Geometry: final body of the model. Coordinates: model frame, mm. A direction names the side the tool comes from. Give positions to 0.01 mm unless a question says otherwise; leave off trailing zeros. Loops run counter-clockwise (first coordinate to the right, second up) from the corner with the lowest first, then second, coordinate; pieces in that order, holes last.
1. Access query for faces 1 (the face through (0, 30, 4)), 2 (the face through (-113.606, 31.364, 8.496)), 3 (the face through (70, 22, 2)). Directions: +Z, -Z, +X, -X, +Y, -Y. A direction counts if a zero-diameter tool reaches every point of the face in a straight line with its end or side. Return the directions, or none.
2. Draft query along Y for faces 4 (the face through (-113.606, 31.364, 1.504)), 5 (the face through (-13.44, 32.25, 6.96)), 6 (the face through (2, 30, 10)), 7 (the face through (-1, 1, 2)). Return one class per face: +Y half, -Y half, draft (parallel to the pull), parting line (faces both ways), or undercut.
3. Section B-B, the plane z = 8.25. Output: boundary loops of the cut face in (x, y), then the cut area to 3 significant figures.
4. Material intervals for line 1 along X through (y, z) = (37.5, 9.5); line 2 along Y through (x, z) = (-70, 6.75); line 3 along X through (y, z) = (43, 3.25), sorted ascending.
5. First-contact query: P1, Ø1.2, axis at x = -70, y = 21.5, coming from the +Z side; P2, Ø2, axis at y = 20.5, z = 1.5, coming from the -X side; P3, Ø1.2, axis at x = -4.5, z = 2, coming from the -Y side; P4, Ø5, axis at x = 12, y = 30, coming from the -Z side. Flat tips, straight axial feed; report the tip coordinate or a pass-through.
from build123d import *

# Parameters (mm, degrees)
BOSS_EXTRUDE1_DEPTH = 10
SKETCH2_R           = 2
CUT_EXTRUDE1_DEPTH  = 8
FILLET1_R           = 5
SKETCH3_W           = 46
SKETCH3_H           = 40
CUT_EXTRUDE2_DEPTH  = 4
SKETCH4_R           = 2.672212582
CUT_EXTRUDE3_DEPTH  = 135.298175803


with BuildPart() as part:
    # Sketch1 → Boss-Extrude1 (new body)
    with BuildSketch(Plane.XY):
        with BuildLine():
            Line((0, 0), (-105, 0))
            ThreePointArc((-105, 0), (-117.249623327, 6.342822149), (-119.139622366, 20.007102889))
            Line((-119.139622366, 20.007102889), (-110.875178831, 43.345171481))
            ThreePointArc((-110.875178831, 43.345171481), (-101.737771304, 55.416038879), (-87.309141554, 60))
            Line((-87.309141554, 60), (87.309141554, 60))
            ThreePointArc((87.309141554, 60), (101.737771304, 55.416038879), (110.875178831, 43.345171481))
            Line((110.875178831, 43.345171481), (119.139622366, 20.007102889))
            ThreePointArc((119.139622366, 20.007102889), (117.249623327, 6.342822149), (105, 0))
            Line((105, 0), (0, 0))
        make_face()
    extrude(amount=BOSS_EXTRUDE1_DEPTH)

    # Sketch2 → Cut-Extrude1 (cut)
    with BuildSketch(Plane.XY.offset(10)):
        with Locations((-70, 22)):
            Circle(SKETCH2_R)
        with Locations((-70, 38)):
            Circle(SKETCH2_R)
        with Locations(Location((70, 22, 0), (0, 0, 180))):
            Circle(SKETCH2_R)
        with Locations(Location((70, 38, 0), (0, 0, 180))):
            Circle(SKETCH2_R)
    extrude(amount=-CUT_EXTRUDE1_DEPTH, mode=Mode.SUBTRACT)

    # Fillet1
    fillet1_edges = [part.edges().sort_by_distance(p)[0] for p in [
        (-117.249623327, 6.342822149, 0),
        (-115.007400599, 31.676137185, 0),
        (-101.737771304, 55.416038879, 0),
        (0, 60, 0),
        (101.737771304, 55.416038879, 0),
        (115.007400599, 31.676137185, 0),
        (117.249623327, 6.342822149, 0),
        (-117.249623327, 6.342822149, 10),
        (-115.007400599, 31.676137185, 10),
        (-101.737771304, 55.416038879, 10),
        (0, 60, 10),
        (101.737771304, 55.416038879, 10),
        (115.007400599, 31.676137185, 10),
        (117.249623327, 6.342822149, 10),
        (0, 0, 0),
        (0, 0, 10),
    ]]
    fillet(fillet1_edges, radius=FILLET1_R - 0.0001)  # a hair under: the kernel refuses the full size

    # Sketch3 → Cut-Extrude2 (cut)
    with BuildSketch(Plane(origin=(0, 0, 0), x_dir=(-1, 0, 0), z_dir=(0, 0, -1))):
        with Locations((0, 30)):
            Rectangle(SKETCH3_W, SKETCH3_H)
    extrude(amount=-CUT_EXTRUDE2_DEPTH, mode=Mode.SUBTRACT)

    # Sketch4 → Cut-Extrude3 (cut, through all)
    with BuildSketch(Plane(origin=(0, 0, 4), x_dir=(-1, 0, 0), z_dir=(0, 0, -1))):
        with Locations((-12, 30)):
            Circle(SKETCH4_R)
        with Locations((12, 30)):
            Circle(SKETCH4_R)
    extrude(amount=-CUT_EXTRUDE3_DEPTH, mode=Mode.SUBTRACT)


solid = part.part
Answers below:
1. face 1: -Z
1. face 2: +Z, -X, +Y
1. face 3: +Z
2. face 4: +Y half
2. face 5: undercut
2. face 6: draft
2. face 7: -Y half
3. outline: (-118.01, 19.61) arc R13.8 ccw to (-105, 1.2) - (105, 1.2) arc R13.8 ccw to (118.01, 19.61) - (109.74, 42.94) arc R23.8 ccw to (87.31, 58.8) - (-87.31, 58.8) arc R23.8 ccw to (-109.74, 42.94) - close; hole circle Ø4 at (-70, 22); hole circle Ø4 at (-70, 38); hole circle Ø5.34 at (-12, 30); hole circle Ø5.34 at (12, 30); hole circle Ø4 at (70, 22); hole circle Ø4 at (70, 38)
3. area: 12,800 mm2
4. line 1: x = -109.95 to -71.94, -68.06 to 68.06, 71.94 to 109.95
4. line 2: y = 0.32 to 20, 24 to 36, 40 to 59.68
4. line 3: x = -110.66 to -23, 23 to 110.66
5. P1: stops at z = 2
5. P2: stops at x = -118.35
5. P3: stops at y = 0.61
5. P4: passes through
